Design review of the part built by this model. Coordinates are the model's own, in mm. Face numbers are marked on the shaded views. A direction names the side the tool comes from. Round coordinates to 2 decimals unless told otherwise and drop trailing zeros. Order: outer loops, then holes, each group sorted by start corner. A loop starts at its lowest first (then second) coordinate and runs counter-clockwise, first axis right, second up. Notation, with made-up numbers: (-31, -25.75) - (7, -25.75) arc R19 ccw to (7, -17.75) - close; hole circle Ø2 at (-25.5, -32.75). An arc over 180 degrees is marked (long way). Write item = value, one per line.
from build123d import *

# Parameters (mm, degrees)
SM_BASE_FLANGE_1_DEPTH      = 40
CUT_EXTRUDE_3_DEPTH         = 10
CUT_EXTRUDE_1_DEPTH         = 92.372862492
SKETCH_7_R                  = 1.6
CUT_EXTRUDE_2_DEPTH         = 92.372862492
SKETCH_9_R                  = 1.65
CUT_EXTRUDE_4_DEPTH         = 93.352585237
PATTERN_LINEAR_1_COUNT      = 2
PATTERN_LINEAR_1_PITCH      = 30
PATTERN_LINEAR_1_COUNT_DIR2 = 2
PATTERN_LINEAR_1_PITCH_DIR2 = 24
FILLET_1_R                  = 5


# Sheet-metal steps are written as plain solids
with BuildPart() as part:
    # Sketch 1 → 基材-凸緣1 (new body)
    with BuildSketch(Plane.XY):
        with BuildLine():
            Line((40, 0), (1, 0))
            ThreePointArc((1, 0), (0.292893219, 0.292893219), (0, 1))
            Line((0, 1), (0, 70))
            Line((0, 70), (-3, 70))
            Line((-3, 70), (-3, 1))
            ThreePointArc((-3, 1), (-1.828427125, -1.828427125), (1, -3))
            Line((1, -3), (40, -3))
            Line((40, -3), (40, 0))
        make_face()
    extrude(amount=SM_BASE_FLANGE_1_DEPTH)

    # 草圖8 → 除料-伸長3 (cut)
    with BuildSketch(Plane.ZY.offset(3)):
        with BuildLine():
            Line((0, 70), (0, 57.002788981))
            ThreePointArc((0, 57.002788981), (8.073899482, 66.465261916), (20, 70))
            Line((20, 70), (0, 70))
        make_face()
        with BuildLine():
            ThreePointArc((20, 70), (31.926100518, 66.465261916), (40, 57.002788981))
            Line((40, 57.002788981), (40, 70))
            Line((40, 70), (20, 70))
        make_face()
    extrude(amount=-CUT_EXTRUDE_3_DEPTH, mode=Mode.SUBTRACT)

    # 草圖6 → 除料-伸長1 (cut, through all)
    with BuildSketch(Plane.ZY.offset(3)):
        with BuildLine():
            Line((26.5, 55.5), (26.5, 41.5))
            ThreePointArc((26.5, 41.5), (20, 35), (13.5, 41.5))
            Line((13.5, 41.5), (13.5, 55.5))
            ThreePointArc((13.5, 55.5), (20, 62), (26.5, 55.5))
        make_face()
    extrude(amount=-CUT_EXTRUDE_1_DEPTH, mode=Mode.SUBTRACT)

    # 草圖7 → 除料-伸長2 (cut, through all)
    with BuildSketch(Plane.ZY.offset(3)):
        with Locations((4.5, 48.5)):
            Circle(SKETCH_7_R)
        with Locations((12.25, 35.076606241)):
            Circle(SKETCH_7_R)
        with Locations((27.75, 35.076606241)):
            Circle(SKETCH_7_R)
        with Locations((35.5, 48.5)):
            Circle(SKETCH_7_R)
        with Locations((27.75, 61.923393759)):
            Circle(SKETCH_7_R)
        with Locations((12.25, 61.923393759)):
            Circle(SKETCH_7_R)
    extrude(amount=-CUT_EXTRUDE_2_DEPTH, mode=Mode.SUBTRACT)

    # 草圖9 → 除料-伸長4 (cut, through all)
    with BuildSketch(Plane.XZ.offset(3)):
        with Locations(Location((32, 35, 0), (0, 0, 270))):
            Circle(SKETCH_9_R)
    cut_extrude_4 = extrude(amount=-CUT_EXTRUDE_4_DEPTH, mode=Mode.SUBTRACT)

    # 直線複製排列1: Cut-Extrude 4 2 × 2
    with Locations(*[(-j * PATTERN_LINEAR_1_PITCH_DIR2, 0, -i * PATTERN_LINEAR_1_PITCH) for i in range(PATTERN_LINEAR_1_COUNT) for j in range(PATTERN_LINEAR_1_COUNT_DIR2) if (i, j) != (0, 0)]):
        add(cut_extrude_4, mode=Mode.SUBTRACT)

    # 圓角1
    fillet_1_edges = [part.edges().sort_by_distance(p)[0] for p in [
        (40, -1.5, 40),
        (40, -1.5, 0),
    ]]
    fillet(fillet_1_edges, radius=FILLET_1_R)


solid = part.part
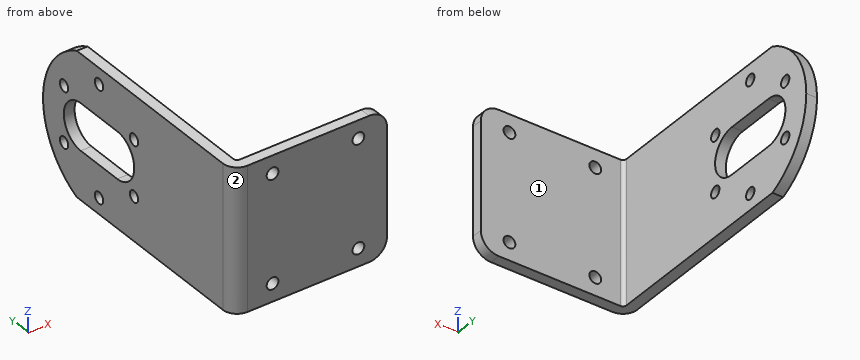
1) We need section D-D on z = 18. Write out the cut boundary in (x, y).
Findings:
outline = (-3, 1) arc R4 ccw to (1, -3) - (40, -3) - (40, 0) - (1, 0) arc R1 cw to (0, 1) - (0, 35.32) - (-3, 35.32) - close; (-3, 61.68) - (0, 61.68) - (0, 69.91) - (-3, 69.91) - close
2) We need section A-A on x = 32. Write out the cut boundary in (y, z).
Findings:
outline = (-3, 0) - (0, 0) - (0, 3.35) - (-3, 3.35) - close; (-3, 6.65) - (0, 6.65) - (0, 33.35) - (-3, 33.35) - close; (-3, 36.65) - (0, 36.65) - (0, 40) - (-3, 40) - close
3) For the marked faces 1 and 2, list the 3-axis set-ups (+Z, -Z, +X, -X, +Y, -Y) from which the entire face can be reached by the end or side of a thin tool; tool diameter is ignored.
Findings:
face_1 = +Z, -Z, +X, +Y
face_2 = +Z, -Z, -X, -Y
4) We need section B-B on z = 27.75. Write out the cut boundary in (x, y), and give its area (3 significant figures).
Findings:
outline = (-3, 1) arc R4 ccw to (1, -3) - (40, -3) - (40, 0) - (1, 0) arc R1 cw to (0, 1) - (0, 33.48) - (-3, 33.48) - close; (-3, 36.68) - (0, 36.68) - (0, 60.32) - (-3, 60.32) - close; (-3, 63.52) - (0, 63.52) - (0, 68.58) - (-3, 68.58) - close
area = 312 mm^2
5) Clearance check with flat-ended pins moving along their axes: pin 1 Ø1.9 at (y, z) = (61.92, 27.75) entering from +X; pin 2 Ø3 at (y, z) = (16.5, 13.5) entering from +X; pin 3 Ø8 at (x, z) = (16, 22.5) entering from +Y. State where each tip first meets the part, or that it passes through.
Findings:
pin_1 = through
pin_2 = 0
pin_3 = 0
6) We need section C-C on y = 48.5. Write out the cut boundary in (x, z).
Findings:
outline = (-3, 0) - (0, 0) - (0, 2.9) - (-3, 2.9) - close; (-3, 6.1) - (0, 6.1) - (0, 13.5) - (-3, 13.5) - close; (-3, 26.5) - (0, 26.5) - (0, 33.9) - (-3, 33.9) - close; (-3, 37.1) - (0, 37.1) - (0, 40) - (-3, 40) - close
7) To check wall thickness, follow L1, parallel to Y at x = -1, z = 12; L2, parallel to X at y = -2.05, z = 5; L3, parallel to X at y = -0.7, z = 35. State the ranges of each line that lie inside material, in increasing order. Write a range as from..to.
Findings:
L1 = -2.46..33.5, 36.66..60.34, 63.5..68.49
L2 = -1.59..6.35, 9.65..30.35, 33.65..40
L3 = -2.62..6.35, 9.65..30.35, 33.65..40
